Drawing for the job (mm, zero at the part's lowest x, y, z). Coordinates: 2 decimals unless noted, no trailing zeros. Order: outer loops, then holes, each group sorted by start corner. A loop starts at its lowest first (then second) coordinate and runs counter-clockwise, first axis right, second up. Notation, with made-up numbers: M -22,13 L 22,13 A26 ccw 22,43 Z; hole C 9.25,-3 d9. An arc over 180 degrees is marked long. Write item = value, one per line. Start each with the question number.
Q1. Band-saw the part on A-A on x = 249. Write the cut outline in (y, z) (1 decimal), plus the area to 3 significant figures.
Q2. Drill centre lines: probe 1 along Z at (x, y) = (229, 0.5) (1 decimal); probe 2 along Z at (x, y) = (279.5, 3.5). Where is each one in solid material? Low to high.
Q3. Band-saw the part on B-B on z = 232. Write the cut outline in (x, y) (1 decimal), plus the area to 3 significant figures.
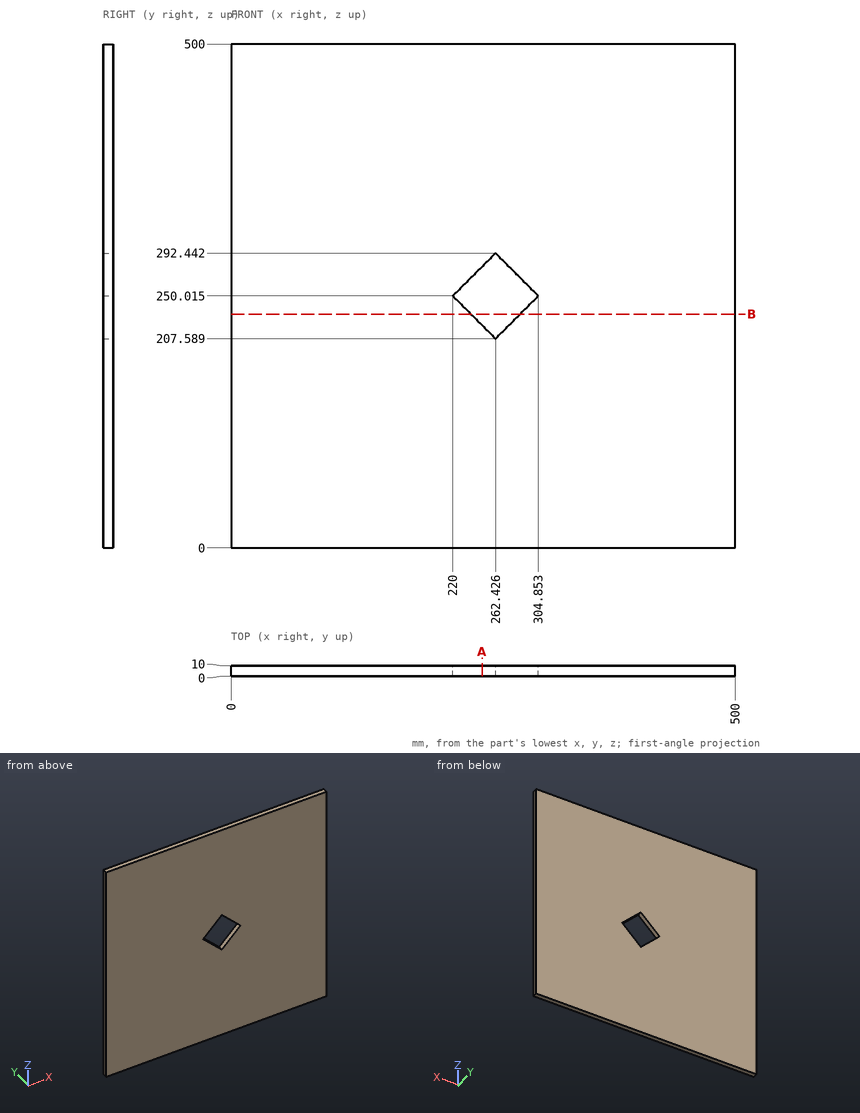
Recorded:
q1.outline = M 0,0 L 10,0 L 10,221 L 0,221 Z; M 0,279 L 10,279 L 10,500 L 0,500 Z
q1.area = 4,420 mm2
q2.probe_1 = 0 to 241, 259 to 500
q2.probe_2 = 0 to 224.66, 275.37 to 500
q3.outline = M 0,0 L 238,0 L 238,10 L 0,10 Z; M 286.8,0 L 500,0 L 500,10 L 286.8,10 Z
q3.area = 4,510 mm2
